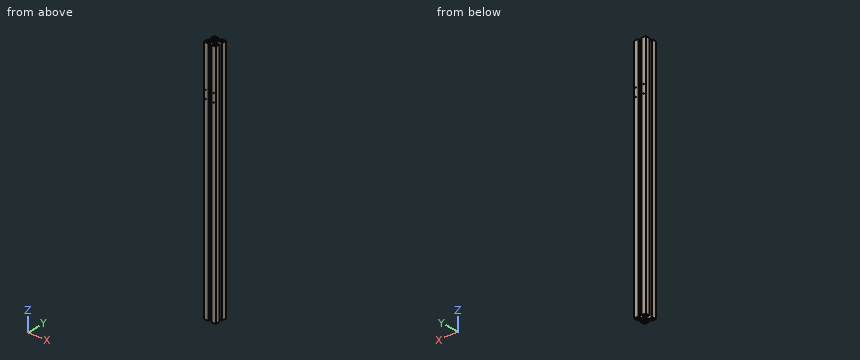
```python
from build123d import *

# Parameters (mm, degrees)
SKETCH_1_W          = 40
SKETCH_1_H          = 40
EXTRUDE_1_DEPTH     = 800
SKETCH_2_R          = 3.25
SKETCH_2_R_2        = 4
CUT_EXTRUDE_1_DEPTH = 801
M3X0_5_1_D          = 2.5
M3X0_5_1_DEPTH      = 7.5
M3X0_5_1_TIP        = 0.751075774
M3X0_5_2_D          = 2.5
M3X0_5_2_DEPTH      = 7.5
M3X0_5_2_TIP        = 0.751075774


with BuildPart() as part:
    # 草圖1 → 伸長1 (new body)
    with BuildSketch(Plane.XY):
        Rectangle(SKETCH_1_W, SKETCH_1_H)
    extrude(amount=EXTRUDE_1_DEPTH)

    # 草圖2 → 除料-伸長1 (cut, through all)
    with BuildSketch(Plane(origin=(0, 0, 0), x_dir=(-1, 0, 0), z_dir=(0, 0, -1))):
        Circle(SKETCH_2_R)
        with Locations((-13.5, 13.5)):
            Circle(SKETCH_2_R_2)
        with Locations((13.5, 13.5)):
            Circle(SKETCH_2_R_2)
        with Locations((-13.5, -13.5)):
            Circle(SKETCH_2_R_2)
        with Locations((13.5, -13.5)):
            Circle(SKETCH_2_R_2)
        with BuildLine():
            Line((5, 14.5), (7.5, 14.5))
            Line((7.5, 14.5), (7.5, 13.5))
            ThreePointArc((7.5, 13.5), (0, 6), (-7.5, 13.5))
            Line((-7.5, 13.5), (-7.5, 14.5))
            Line((-7.5, 14.5), (-5, 14.5))
            Line((-5, 14.5), (-5, 20))
            Line((-5, 20), (5, 20))
            Line((5, 20), (5, 14.5))
        make_face()
        with BuildLine():
            Line((14.5, -5), (14.5, -7.5))
            Line((14.5, -7.5), (13.5, -7.5))
            ThreePointArc((13.5, -7.5), (6, 0), (13.5, 7.5))
            Line((13.5, 7.5), (14.5, 7.5))
            Line((14.5, 7.5), (14.5, 5))
            Line((14.5, 5), (20, 5))
            Line((20, 5), (20, -5))
            Line((20, -5), (14.5, -5))
        make_face()
        with BuildLine():
            Line((-5, -14.5), (-7.5, -14.5))
            Line((-7.5, -14.5), (-7.5, -13.5))
            ThreePointArc((-7.5, -13.5), (0, -6), (7.5, -13.5))
            Line((7.5, -13.5), (7.5, -14.5))
            Line((7.5, -14.5), (5, -14.5))
            Line((5, -14.5), (5, -20))
            Line((5, -20), (-5, -20))
            Line((-5, -20), (-5, -14.5))
        make_face()
        with BuildLine():
            Line((-14.5, 5), (-14.5, 7.5))
            Line((-14.5, 7.5), (-13.5, 7.5))
            ThreePointArc((-13.5, 7.5), (-6, 0), (-13.5, -7.5))
            Line((-13.5, -7.5), (-14.5, -7.5))
            Line((-14.5, -7.5), (-14.5, -5))
            Line((-14.5, -5), (-20, -5))
            Line((-20, -5), (-20, 5))
            Line((-20, 5), (-14.5, 5))
        make_face()
    extrude(amount=-CUT_EXTRUDE_1_DEPTH, mode=Mode.SUBTRACT)

    # M3x0.5 螺紋孔1
    with Locations(Plane(origin=(0, 20, 0), x_dir=(1, 0, 0), z_dir=(0, 1, 0))):
        with Locations((13.5, -663.5), (13.5, -636.5), (-13.5, -636.5), (-13.5, -663.5)):
            Hole(M3X0_5_1_D / 2, depth=M3X0_5_1_DEPTH)
            with Locations((0, 0, -(M3X0_5_1_DEPTH + M3X0_5_1_TIP / 2))):  # 118° drill point
                Cone(0, M3X0_5_1_D / 2, M3X0_5_1_TIP, mode=Mode.SUBTRACT)

    # M3x0.5 螺紋孔2
    with Locations(Plane(origin=(0, -20, 0), x_dir=(-1, 0, 0), z_dir=(0, -1, 0))):
        with Locations((13.5, -636.5), (13.5, -663.5), (-13.5, -663.5), (-13.5, -636.5)):
            Hole(M3X0_5_2_D / 2, depth=M3X0_5_2_DEPTH)
            with Locations((0, 0, -(M3X0_5_2_DEPTH + M3X0_5_2_TIP / 2))):  # 118° drill point
                Cone(0, M3X0_5_2_D / 2, M3X0_5_2_TIP, mode=Mode.SUBTRACT)


solid = part.part
```
Could you check a few things on this model? Use its own coordinates, in mm. Give positions to 0.01 mm unless a question says otherwise; leave off trailing zeros. One line per item, written item: value. Start each with the question number.
Item 1: Please list where these lines run through material, in increasing order: line 1 (Z direction, x = 13, y = 19); line 2 (Z direction, x = -13.5, y = -18.8); line 3 (Y direction, x = 14, z = 670). Write a range as from..to.
Item 2: I'm going to push flat-ended pins straight in: pin 1 (4 mm diameter, centred on x = 1, z = 621.5, fed in from -Y); pin 2 (10.5 mm diameter, centred on x = 13.5, y = -13.5, fed in from +Z); pin 3 (2 mm diameter, centred on x = -13.5, z = 663.5, fed in from -Y). Where does each tip first touch, or does it pass through?
Item 3: Imagine slicing it at A-A, the plane z = 366.5. Give the number of separate pieces and of enclosed holes in the cut face, and give its area (3 significant figures).
Geometry says:
1. line 1: 0..635.35, 637.65..662.35, 664.65..800
1. line 2: 0..635.25, 637.75..662.25, 664.75..800
1. line 3: -20..-17.47, -9.53..-7.5, 7.5..9.53, 17.47..20
2. pin 1: y = -6.63
2. pin 2: z = 800
2. pin 3: y = -9.63
3. separate pieces: 1
3. enclosed holes: 5
3. area: 732 mm^2
